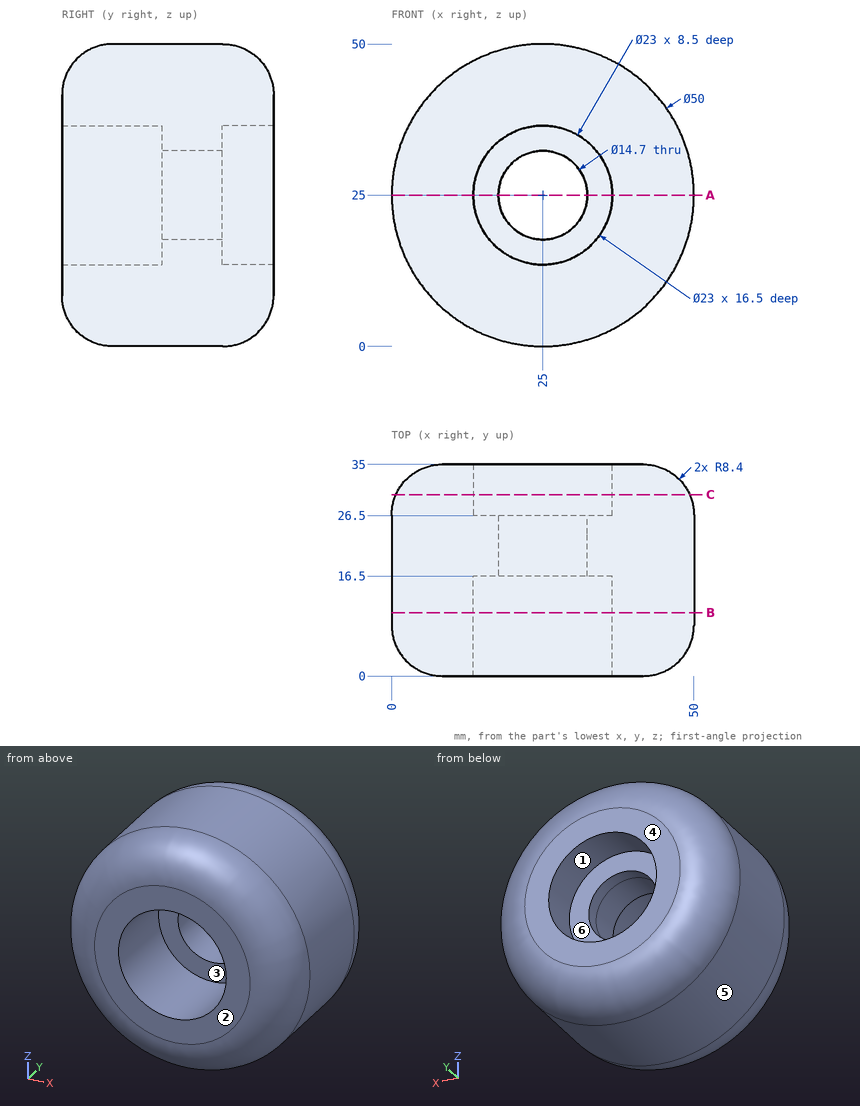
Design review of the part shown in the three views and the two pictorial views. Dimensions are in mm from the part's minimum x, y and z. A direction names the side the tool comes from. Round coordinates to 2 decimals unless told otherwise and drop trailing zeros. Write each loop counter-clockwise with the first axis right and the second up, starting at its lowest first coordinate (ties: lowest second). Pieces come first, ordered by that corner, then holes. Notation, with made-up numbers: (75, 3) - (94, 3) arc R15 cw to (94, 20) - close; hole circle Ø8 at (80.25, 50.5). An arc over 180 degrees is marked (long way). Return JSON: item names as keys, results as strings. Group by question number.
Item 1: Machinability: for the marked faces 1, 2 and 3, which of the approach directions +Z, -Z, +X, -X, +Y, -Y give a long, thin tool a straight path to every point of the face, cutting with its end or side? Answer none if there is none.
Item 2: We need section B-B on y = 10.5. Write out the cut boundary in (x, z).
Item 3: The part is to be moulded in two halves that separate along Z. For the marked faces 4, 5 and 6, say which applies: pulls with the +Z half, pulls with the -Z half, needs draft (parallel to the pull), parting line crosses it, or undercut.
Item 4: We need section C-C on y = 30. Write out the cut boundary in (x, z), and give its area (3 significant figures).
Item 5: Insertion check: P1, Ø20.5, axis at x = 25, z = 25, coming from the +Y side; P2, Ø8, axis at x = 42, z = 8, coming from the -Y side; P3, Ø1.5, axis at y = 26, z = 14.5, coming from the -X side. Each pin has a flat end and moves straight along its axis. Give the tip position at first contact, or say it passes through.
Item 6: For probe 1 along Z at (x, y) = (25, 25.4); probe 2 along Z at (x, y) = (24.5, 16) (3 decimals); probe 3 along Y at (x, z) = (9, 30.5), list the stretches that pass through material, from the lowest coordinate up. Write a range as [from, to].
Item 7: We need section A-A on z = 25. Write out the cut boundary in (x, y), and give its area (3 significant figures).
Model answer:
{
 "1": {"face 1": "+Y", "face 2": "+Z, -Z, +X, -X, -Y", "face 3": "-Y"},
 "2": {"outline": "circle Ø50 at (25, 25); hole circle Ø23 at (25, 25)"},
 "3": {"face 4": "needs draft", "face 5": "parting line crosses it", "face 6": "undercut"},
 "4": {"outline": "circle Ø48.56 at (25, 25); hole circle Ø23 at (25, 25)", "area": "1,440 mm²"},
 "5": {"P1": "stops at y = 26.5", "P2": "stops at y = 0.74", "P3": "stops at x = 1.98"},
 "6": {"probe 1": "z = [0, 17.65], [32.35, 50]", "probe 2": "z = [0.005, 13.511], [36.489, 49.995]", "probe 3": "y = [0.01, 34.99]"},
 "7": {"outline": "(0, 8.4) arc R8.4 ccw to (8.4, 0) - (13.5, 0) - (13.5, 16.5) - (17.65, 16.5) - (17.65, 26.5) - (13.5, 26.5) - (13.5, 35) - (8.4, 35) arc R8.4 ccw to (0, 26.6) - close; (32.35, 16.5) - (36.5, 16.5) - (36.5, 0) - (41.6, 0) arc R8.4 ccw to (50, 8.4) - (50, 26.6) arc R8.4 ccw to (41.6, 35) - (36.5, 35) - (36.5, 26.5) - (32.35, 26.5) - close", "area": "967 mm²"}
}
